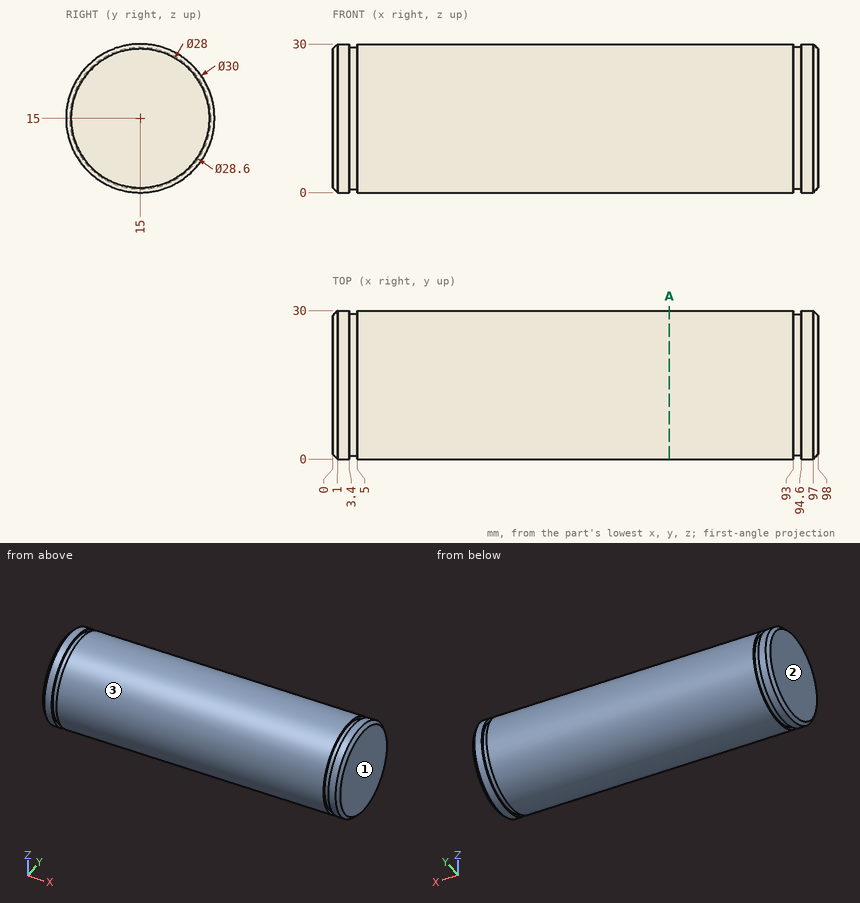
Geometry: see drawing. Coordinates: mm, zero at the bounding-box minimum. Round coordinates to 2 decimals unless told otherwise and drop trailing zeros. Write each loop counter-clockwise with the first axis right and the second up, starting at its lowest first coordinate (ties: lowest second). Pieces come first, ordered by that corner, then holes. Notation, with made-up numbers: M 69,-1.75 L 124,-1.75 A16 cw 124,29.25 Z; hole C -32,80 d6. An arc over 180 degrees is marked long. Answer in a Markdown table with one row per item. Add a question column.
(1) Contact query for flat-ended pins moving along their axis: pin 1 (6 mm diameter, centred on x = 19.5, y = 11, fed in from +Z); pin 2 (12 mm diameter, centred on x = 45.5, y = 6.5, fed in from -Z); pin 3 (8 mm diameter, centred on x = 64.5, z = 5.5, fed in from +Y). Output: stop coordinate, or through.
(2) Draft query along X for the marked faces 1, 2 and 3. Return one class per face: pulls with the +X half, pulls with the -X half, needs draft (parallel to the pull), parting line crosses it, or undercut.
(3) Ray query, L1, parallel to Z at x = 17, y = 15.25; L2, parallel to Z at x = 31.5, y = 10.5; L3, parallel to Y at x = 74, z = 4.25. Return the intervals inside material, ascending.
(4) Cut plane A-A, the plane x = 68. Return the cut outline in (y, z), then the cut area to 3 significant figures.
Established:
| question | item | result |
|---|---|---|
| 1 | pin 1 | z = 29.97 |
| 1 | pin 2 | z = 0.21 |
| 1 | pin 3 | y = 28.96 |
| 2 | face 1 | pulls with the +X half |
| 2 | face 2 | pulls with the -X half |
| 2 | face 3 | needs draft |
| 3 | L1 | 0 to 30 |
| 3 | L2 | 0.69 to 29.31 |
| 3 | L3 | 4.54 to 25.46 |
| 4 | outline | C 15,15 d30 |
| 4 | area | 707 mm² |
